```python
from build123d import *

# Parameters (mm, degrees)
F0_R     = 21.4249
F0_R_2   = 15.367
F1_DEPTH = 20.066
F2_R     = 15.367
F3_DEPTH = 32.512
F4_SIZE2 = 0.127
F4_SIZE  = 0.127


with BuildPart() as f1:
    # F0 (on Front) → F1 (new body)
    with BuildSketch(Plane.XZ):
        Circle(F0_R)
        Circle(F0_R_2, mode=Mode.SUBTRACT)
        Circle(F0_R_2)
    extrude(amount=F1_DEPTH)

    # F2 (on Front) → F3 (join)
    with BuildSketch(Plane.XZ):
        Circle(F2_R)
    extrude(amount=F3_DEPTH)

    # F4
    f4_edges = [f1.edges().sort_by_distance(p)[0] for p in [
        (-15.367, -32.512, 0),
    ]]
    chamfer(f4_edges, length=F4_SIZE, length2=F4_SIZE2)


solid = f1.part
```
Model file for the job. Use its own axes, mm. A direction names the side the tool comes from. Coordinates: 2 decimals unless noted, no trailing zeros. Order: outer loops, then holes, each group sorted by start corner. A loop starts at its lowest first (then second) coordinate and runs counter-clockwise, first axis right, second up. Notation, with made-up numbers: (-9.5, -27.5) -> (49.5, -27.5) arc R18 cw to (49.5, 1.5) -> close; hole circle Ø2 at (19, 8). An arc over 180 degrees is marked (long way). Return JSON: item names as keys, results as strings.
Item 1: Slice it at A-A (x = 0). Write the cut outline in (y, z) (3 decimals).
Model answer:
{"outline": "(-32.512, -15.24) -> (-32.385, -15.367) -> (-20.066, -15.367) -> (-20.066, -21.425) -> (0, -21.425) -> (0, 21.425) -> (-20.066, 21.425) -> (-20.066, 15.367) -> (-32.385, 15.367) -> (-32.512, 15.24) -> close"}
Item 2: Wall check: line 1 along Y through (x, z) = (18, 10.5); line 2 along X through (y, z) = (-12, 17.5); line 3 along Z through (x, y) = (-12.5, -8.5). Give the ranges that are in metal, low to high. Write a range as from..to.
Model answer:
{"line 1": "y = -20.07..0", "line 2": "x = -12.36..12.36", "line 3": "z = -17.4..17.4"}
Item 3: 3-axis set-ups, long thin cutter, end or side, ignore diameter. For faces 1 (the face through (0, -32.512, 0)), 2 (the face through (14.657, -26.139, 4.616)): which of +Z, -Z, +X, -X, +Y, -Y reach the whole face in a straight line?
Model answer:
{"face 1": "+Z, -Z, +X, -X, -Y", "face 2": "-Y"}
Item 4: Pin check, flat tips, straight feed: P1, Ø1.5, axis at x = 15, z = -10, coming from the +Y side; P2, Ø1, axis at x = 15, y = -11, coming from the -Z side; P3, Ø12, axis at x = -1, y = -5, coming from the -Z side; P4, Ø4, axis at x = -9, y = -28, coming from the -Z side. Stop position of each tip, or through.
Model answer:
{"P1": "stops at y = 0", "P2": "stops at z = -15.77", "P3": "stops at z = -21.42", "P4": "stops at z = -13.68"}
Item 5: Slice it at B-B (z = 0). Write the cut outline in (x, y) (3 decimals).
Model answer:
{"outline": "(-21.425, -20.066) -> (-15.367, -20.066) -> (-15.367, -32.385) -> (-15.24, -32.512) -> (15.24, -32.512) -> (15.367, -32.385) -> (15.367, -20.066) -> (21.425, -20.066) -> (21.425, 0) -> (-21.425, 0) -> close"}
Item 6: Slice it at C-C (y = -11.5). Write the cut outline in (x, z).
Model answer:
{"outline": "circle Ø42.85 at (0, 0)"}
Item 7: Slice it at D-D (y = -30). Write the cut outline in (x, z), then the cut area to 3 significant figures.
Model answer:
{"outline": "circle Ø30.73 at (0, 0)", "area": "742 mm²"}
